Verification items for the finished model (mm, model axes). Coordinates: 2 decimals unless noted, no trailing zeros. Order: outer loops, then holes, each group sorted by start corner. A loop starts at its lowest first (then second) coordinate and runs counter-clockwise, first axis right, second up. Notation, with made-up numbers: (-9, 66.25) -> (26, 66.25) arc R21 ccw to (26, 92.25) -> close; hole circle Ø7 at (48.25, 9.5). An arc over 180 degrees is marked (long way). Write item = value, one per line. Start each with the question number.
1. Cross-section at D-D on y = -2. Record the cut outline in (x, z), plus the area to 3 significant figures.
2. Cross-section at C-C on x = 0. Record the cut outline in (y, z) (3 decimals), plus the area to 3 significant figures.
3. Cross-section at A-A on x = -26.5. Record the cut outline in (y, z).
4. Thickness scan on line 1 along Y through (x, z) = (-18.5, -0.1); line 2 along Y through (x, z) = (0, -0.15) (3 decimals); line 3 along X through (y, z) = (-2.75, -0.15). Record the ranges inside material, lowest first. Write a range as from..to.
5. Go/stop test with a flat-tipped pin: P1, Ø5, axis at x = 0, y = 0, coming from the -Z side. Record where the tip stops, or that it passes through.
6. Cross-section at B-B on z = 0.4. Give the number of separate pieces and of enclosed holes in the cut face, plus the area to 3 significant figures.
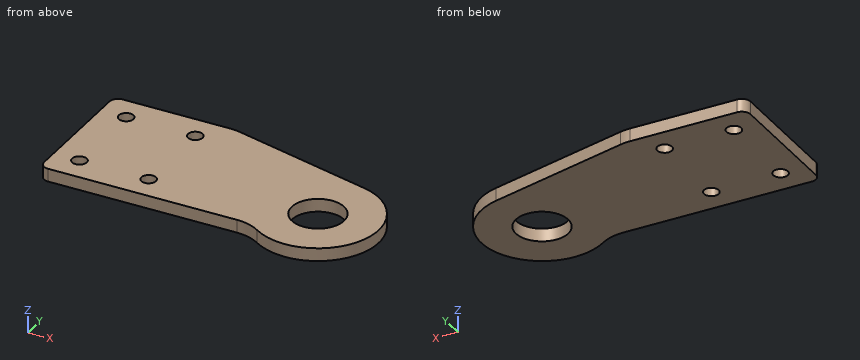
from build123d import *

# Parameters (mm, degrees)
ESQUISSE1_R        = 3.025
ESQUISSE1_R_2      = 0.85
BOSS_EXTRU_1_DEPTH = 0.75
CONG_1_R           = 5
CONG_2_R           = 1


with BuildPart() as part:
    # Esquisse1 → Boss.-Extru.1 (new body, symmetric)
    with BuildSketch(Plane.XY):
        with BuildLine():
            Line((-15.5, 11), (1.660328935, 6.825974863))
            ThreePointArc((1.660328935, 6.825974863), (6.135445446, -3.421539739), (-4.934635245, -5))
            Line((-4.934635245, -5), (-15.5, -5))
            Line((-15.5, -5), (-29.5, -5))
            Line((-29.5, -5), (-29.5, 11))
            Line((-29.5, 11), (-15.5, 11))
        make_face()
        Circle(ESQUISSE1_R, mode=Mode.SUBTRACT)
        with Locations((-26.5, 8)):
            Circle(ESQUISSE1_R_2, mode=Mode.SUBTRACT)
        with Locations((-18.5, 8)):
            Circle(ESQUISSE1_R_2, mode=Mode.SUBTRACT)
        with Locations((-18.5, -2)):
            Circle(ESQUISSE1_R_2, mode=Mode.SUBTRACT)
        with Locations((-26.5, -2)):
            Circle(ESQUISSE1_R_2, mode=Mode.SUBTRACT)
    extrude(amount=BOSS_EXTRU_1_DEPTH, both=True)

    # Congé1
    cong_1_edges = [part.edges().sort_by_distance(p)[0] for p in [
        (-15.5, 11, 0),
        (-4.934635245, -5, 0),
    ]]
    fillet(cong_1_edges, radius=CONG_1_R)

    # Congé2
    cong_2_edges = [part.edges().sort_by_distance(p)[0] for p in [
        (-29.5, 11, 0),
        (-29.5, -5, 0),
    ]]
    fillet(cong_2_edges, radius=CONG_2_R)


solid = part.part
Worked out:
q1.outline = (-29.5, -0.75) -> (-27.35, -0.75) -> (-27.35, 0.75) -> (-29.5, 0.75) -> close; (-25.65, -0.75) -> (-19.35, -0.75) -> (-19.35, 0.75) -> (-25.65, 0.75) -> close; (-17.65, -0.75) -> (-2.27, -0.75) -> (-2.27, 0.75) -> (-17.65, 0.75) -> close; (2.27, -0.75) -> (6.73, -0.75) -> (6.73, 0.75) -> (2.27, 0.75) -> close
q1.area = 42.4 mm²
q2.outline = (-7.025, -0.75) -> (-3.025, -0.75) -> (-3.025, 0.75) -> (-7.025, 0.75) -> close; (3.025, -0.75) -> (7.23, -0.75) -> (7.23, 0.75) -> (3.025, 0.75) -> close
q2.area = 12.3 mm²
q3.outline = (-5, -0.75) -> (-2.85, -0.75) -> (-2.85, 0.75) -> (-5, 0.75) -> close; (-1.15, -0.75) -> (7.15, -0.75) -> (7.15, 0.75) -> (-1.15, 0.75) -> close; (8.85, -0.75) -> (11, -0.75) -> (11, 0.75) -> (8.85, 0.75) -> close
q4.line_1 = -5..-2.85, -1.15..7.15, 8.85..11
q4.line_2 = -7.025..-3.025, 3.025..7.23
q4.line_3 = -29.5..-26.9, -26.1..-18.9, -18.1..-1.26, 1.26..6.46
q5.P1 = through
q6.separate_pieces = 1
q6.enclosed_holes = 5
q6.area = 489 mm²
